Part model, mm, in its own coordinate system. Coordinates: 2 decimals unless noted, no trailing zeros. Order: outer loops, then holes, each group sorted by start corner. A loop starts at its lowest first (then second) coordinate and runs counter-clockwise, first axis right, second up.
```python
from build123d import *

# Parameters (mm, degrees)
ESQUISSE1_W       = 250
ESQUISSE1_H       = 250
EXTRUSION1_DEPTH  = 3
EXTRUSION11_DEPTH = 13


with BuildPart() as part:
    # Esquisse1 → Extrusion1 (new body)
    with BuildSketch(Plane(origin=(0, 0, 0), x_dir=(1, 0, 0), z_dir=(0, 1, 0))):
        Rectangle(ESQUISSE1_W, ESQUISSE1_H)
    extrude(amount=EXTRUSION1_DEPTH)

    # Esquisse2 → Extrusion11 (cut)
    with BuildSketch(Plane(origin=(0, 3, 0), x_dir=(1, 0, 0), z_dir=(0, 1, 0))):
        Polygon((-125, 125), (-125, 65), (-65, 125), align=None)
        Polygon((125, 125), (65, 125), (125, 65), align=None)
        Polygon((125, -65), (65, -125), (125, -125), align=None)
        Polygon((-65, -125), (-125, -65), (-125, -125), align=None)
    extrude(amount=-EXTRUSION11_DEPTH, mode=Mode.SUBTRACT)


solid = part.part
```
(1) Drop a flat-ended pin along its axis: pin 1 (1 mm diameter, centred on x = 82.5, y = 0.5, fed in from +Z). Give the stop position or say it passes through.
(2) Slice it at B-B, the plane x = -68. Give the cut face in (y, z).
(3) Probe line 1 (X direction, y = 1.9, z = -108.5); line 2 (X direction, y = 2.85, z = -111.5); line 3 (Z direction, x = -113.5, y = 1.9). List the from-to ranges inside material, lowest first.
(4) Slice it at A-A, the plane y = 1.95. Give the cut face in (x, z), then the cut area to 3 significant figures.
(5) Slice it at C-C, the plane z = 94.5. Give the cut face in (x, y), then the cut area to 3 significant figures.
Here are the results:
1. pin 1: stops at z = 108
2. outline: (0, -122) - (3, -122) - (3, 122) - (0, 122) - close
3. line 1: x = -81.5 to 81.5
3. line 2: x = -78.5 to 78.5
3. line 3: z = -76.5 to 76.5
4. outline: (-125, -65) - (-65, -125) - (65, -125) - (125, -65) - (125, 65) - (65, 125) - (-65, 125) - (-125, 65) - close
4. area: 55,300 mm2
5. outline: (-95.5, 0) - (95.5, 0) - (95.5, 3) - (-95.5, 3) - close
5. area: 573 mm2
